For this review, take the finished solid that the model builds, in its own axes (mm). Face numbers are marked on the shaded views. A direction names the side the tool comes from. Give positions to 0.01 mm unless a question says otherwise; leave off trailing zeros. Order: outer loops, then holes, each group sorted by start corner. A loop starts at its lowest first (then second) coordinate and runs counter-clockwise, first axis right, second up. Notation, with made-up numbers: M 12.5,55.25 L 28.5,55.25 A27 cw 28.5,82.25 Z; hole C 29.5,-6 d5. An arc over 180 degrees is marked long. Use CSV: the item, a comma, the result in double quotes. Start each with the question number.
(1) Consider section C-C (y = 0). Write out the cut boundary in (x, z), and give its area (3 significant figures).
(2) Consider section B-B (z = -35). Write out the cut boundary in (x, y).
(3) Wall thickness on L1, parallel to Y at x = -30, z = -75; L2, parallel to Y at x = -0.5, z = -29.5; L3, parallel to Y at x = -25, z = -75.25: over which ranges is each line inside the solid? List them lowest first. Write a range as from..to.
(4) Tool access review of the marked faces 1 and 2: name each direction out of +Z, -Z, +X, -X, +Y, -Y from which nothing blocks a thin tool from reaching the whole face with its end or side.
(5) Clearance check with flat-ended pins moving along their axes: P1, Ø15.5, axis at y = -59, z = -33.13, coming from the -X side; P2, Ø3, axis at x = -31.5, y = -42.5, coming from the +Z side. State where each tip first meets the part, or that it passes through.
(6) Consider section A-A (y = -61). Write out the cut boundary in (x, z), and give its area (3 significant figures).
(7) Consider section D-D (x = -40). Write out the cut boundary in (y, z).
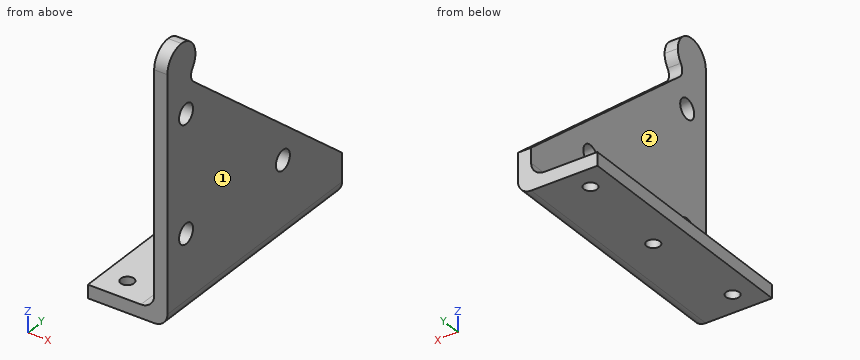
```python
from build123d import *

# Parameters (mm, degrees)
F1_DEPTH = 75
F2_R     = 8
F3_R     = 6
F4_DEPTH = 48.001
F5_R     = 4
F6_DEPTH = 80.001


with BuildPart() as f1:
    # F0 (on Front) → F1 (new body, symmetric)
    with BuildSketch(Plane.XZ):
        Polygon((4, 80), (-4, 80), (-4, -72), (-44, -72), (-44, -80), (4, -80), align=None)
    extrude(amount=F1_DEPTH, both=True)

    # F2
    f2_edges = [f1.edges().sort_by_distance(p)[0] for p in [
        (-4, 0, -72),
        (4, 0, -80),
    ]]
    fillet(f2_edges, radius=F2_R)

    # F3 (on face) → F4 (cut, through all)
    with BuildSketch(Plane.YZ.offset(4)):
        with BuildLine():
            ThreePointArc((-63, 80), (-54.514719, 76.485281), (-51, 68))
            ThreePointArc((-51, 68), (-51.64257, 64.125884), (-53.501462, 60.666667))
            ThreePointArc((-53.501462, 60.666667), (-54.717975, 56.360123), (-52.61582, 52.409533))
            Line((-52.61582, 52.409533), (75, -55))
            Line((75, -55), (75, 80))
            Line((75, 80), (-63, 80))
        make_face()
        with BuildLine():
            ThreePointArc((-75, 68), (-71.485281, 76.485281), (-63, 80))
            Line((-63, 80), (-75, 80))
            Line((-75, 80), (-75, 68))
        make_face()
        with Locations((-59, 36.869957)):
            Circle(F3_R)
        with Locations((-59, -33.130043)):
            Circle(F3_R)
        with Locations((24.168664, -33.130043)):
            Circle(F3_R)
    extrude(amount=-F4_DEPTH, mode=Mode.SUBTRACT)

    # F5 (on Top) → F6 (cut, through all)
    with BuildSketch(Plane.XY):
        with Locations((-30, -61)):
            Circle(F5_R)
        with Locations((-25, 0)):
            Circle(F5_R)
        with Locations((-30, 61)):
            Circle(F5_R)
    extrude(amount=-F6_DEPTH, mode=Mode.SUBTRACT)


solid = f1.part
```
Check result:
1,outline,"M -44,-80 L -29,-80 L -29,-72 L -44,-72 Z; M -21,-80 L -4,-80 A8 ccw 4,-72 L 4,8.12 L -4,8.12 L -4,-64 A8 cw -12,-72 L -21,-72 Z"
1,area,"961 mm^2"
2,outline,"M -4,-75 L 4,-75 L 4,-64.7 L -4,-64.7 Z; M -4,-53.3 L 4,-53.3 L 4,18.47 L -4,18.47 Z; M -4,29.87 L 4,29.87 L 4,51.24 L -4,51.24 Z"
3,L1,"y = -75..-65, -57..57, 65..75"
3,L2,"y = -75..-63.78, -54.22..19.39, 28.95..44.7"
3,L3,"y = -75..-4, 4..75"
4,face 1,"+Z, -Z, +X, +Y, -Y"
4,face 2,"+Z, -X, +Y, -Y"
5,P1,"stops at x = -4"
5,P2,"stops at z = -72"
6,outline,"M -44,-80 L -34,-80 L -34,-72 L -44,-72 Z; M -26,-80 L -4,-80 A8 ccw 4,-72 L 4,-38.79 L -4,-38.79 L -4,-64 A8 cw -12,-72 L -26,-72 Z; M -4,-27.47 L 4,-27.47 L 4,31.21 L -4,31.21 Z; M -4,42.53 L 4,42.53 L 4,79.83 L -4,79.83 Z"
6,area,"1,350 mm^2"
7,outline,"M -75,-80 L 75,-80 L 75,-72 L -75,-72 Z"
